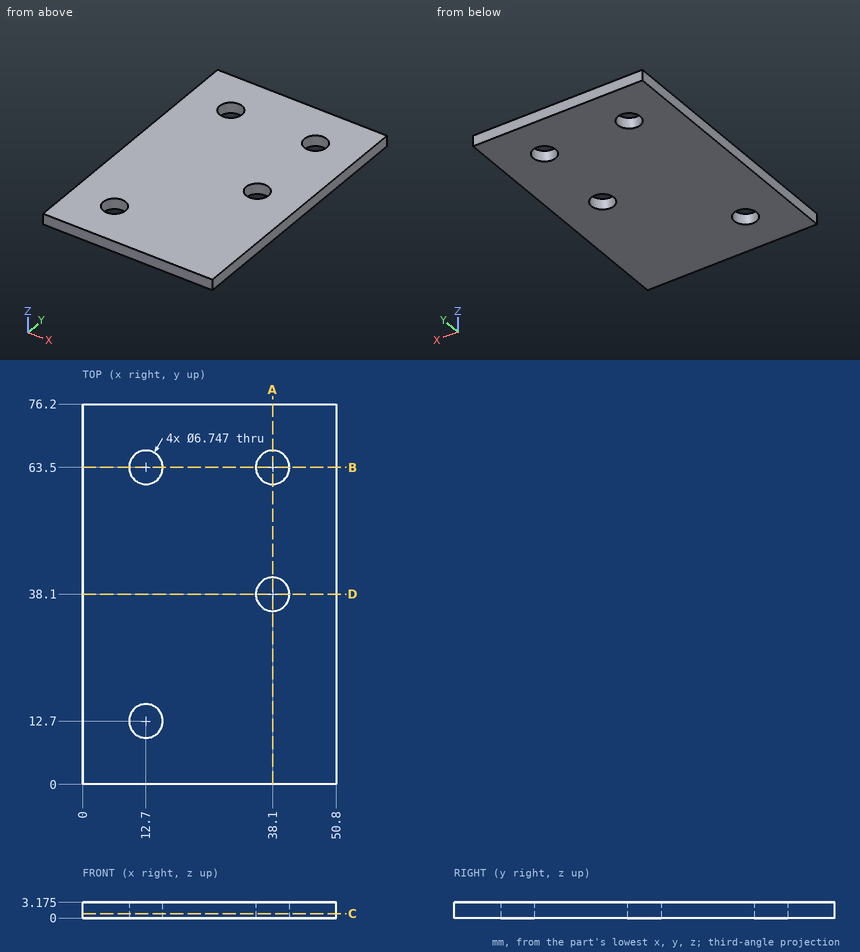
Can you work these out from the drawing? Everything is in mm from the part's minimum corner. Coordinates: 2 decimals unless noted, no trailing zeros. Write each loop counter-clockwise with the first axis right and the second up, starting at its lowest first coordinate (ties: lowest second). Pieces come first, ordered by that corner, then holes. Notation, with made-up numbers: (-28, 43.25) -> (-3, 43.25) arc R15 cw to (-3, 71.25) -> close; hole circle Ø9 at (5.5, 89.5). An arc over 180 degrees is marked (long way). Write each question's results on one line, items separated by ' | '. Start each with the question number.
Item 1: If we section it at B-B, the plane y = 63.5: Write out the boundary of the cut face in (x, z) (1 decimal), and give its area (3 significant figures).
Item 2: If we section it at D-D, the plane y = 38.1: Write out the boundary of the cut face in (x, z) (1 decimal), and give its area (3 significant figures).
Item 3: If we section it at A-A, the plane x = 38.1: Write out the boundary of the cut face in (y, z) (1 decimal).
Item 4: Please list where these lines run through material, in increasing order: probe 1 along Y at (x, z) = (12.7, 2.3); probe 2 along Y at (x, z) = (38.1, 0.7); probe 3 along X at (y, z) = (11.5, 2.6).
Item 5: If we section it at C-C, the plane z = 0.95: Write out the boundary of the cut face in (x, y).
Answer block:
1) outline: (0, 0) -> (9.3, 0) -> (9.3, 3.2) -> (0, 3.2) -> close; (16.1, 0) -> (34.7, 0) -> (34.7, 3.2) -> (16.1, 3.2) -> close; (41.5, 0) -> (50.8, 0) -> (50.8, 3.2) -> (41.5, 3.2) -> close | area: 118 mm²
2) outline: (0, 0) -> (34.7, 0) -> (34.7, 3.2) -> (0, 3.2) -> close; (41.5, 0) -> (50.8, 0) -> (50.8, 3.2) -> (41.5, 3.2) -> close | area: 140 mm²
3) outline: (0, 0) -> (34.7, 0) -> (34.7, 3.2) -> (0, 3.2) -> close; (41.5, 0) -> (60.1, 0) -> (60.1, 3.2) -> (41.5, 3.2) -> close; (66.9, 0) -> (76.2, 0) -> (76.2, 3.2) -> (66.9, 3.2) -> close
4) probe 1: 0 to 9.33, 16.07 to 60.13, 66.87 to 76.2 | probe 2: 0 to 34.73, 41.47 to 60.13, 66.87 to 76.2 | probe 3: 0 to 9.55, 15.85 to 50.8
5) outline: (0, 0) -> (50.8, 0) -> (50.8, 76.2) -> (0, 76.2) -> close; hole circle Ø6.75 at (12.7, 12.7); hole circle Ø6.75 at (12.7, 63.5); hole circle Ø6.75 at (38.1, 38.1); hole circle Ø6.75 at (38.1, 63.5)
